Could you check a few things on this model? Use its own coordinates, in mm. Give positions to 0.01 mm unless a question says otherwise; leave off trailing zeros. Loops run counter-clockwise (first coordinate to the right, second up) from the corner with the lowest first, then second, coordinate; pieces in that order, holes last. Notation, with made-up numbers: (42, 23.25) -> (68, 23.25) arc R12 cw to (68, 29.25) -> close; hole circle Ø6 at (88.25, 23.25). An arc over 180 degrees is marked (long way). Write item = value, one per line. Start each with the question number.
1) I want a section at B-B (x = 35). List the corners of the cut face in (y, z) for me.
2) I'm going to push flat-ended pins straight in: pin 1 Ø4 at (y, z) = (167.5, 12) entering from +X; pin 2 Ø10 at (x, y) = (14.5, 78.5) entering from -Z; pin 3 Ø3 at (y, z) = (142.5, 20) entering from -X. Where does each tip first touch, or does it pass through?
3) I want a section at C-C (y = 74.5). List the corners of the cut face in (x, z) for me, and give its area (3 significant figures).
4) If we mould it in two halves opening along X, with no side actions, what happens to faces 1 (the face through (-10.84, 98.6, 48.81)), 2 (the face through (-34, 0, 33)), 3 (the face through (-21.68, 144.19, -42.03))? For each: +X half, -X half, draft (parallel to the pull), parting line (faces both ways), or undercut.
5) I want a section at A-A (z = 0). List the corners of the cut face in (x, y) for me.
6) I need wall thicknesses on probe 1 along X at (y, z) = (125, 0); probe 2 along Z at (x, y) = (0, 144). Which ranges of each line are inside material? Lowest first, please. Write a range as from..to.
from build123d import *

# Parameters (mm, degrees)
EXTRUDE_1_OUTLINE_R      = 50
EXTRUDE_1_OUTLINE_R_2    = 47
EXTRUDE_1_DEPTH          = 200
CUT_EXTRUDE_1_DEPTH      = 213.132034356
CUT_EXTRUDE_1_DEPTH_BACK = 213.132034356
SKETCH_2_R               = 66.5


# Read off the part's stored shape, not the designer's step: Вытянуть-Тонкостенный1
with BuildPart() as part:
    # Вытянуть-Тонкостенный1 outline → Вытянуть-Тонкостенный1 (new body)
    with BuildSketch(Plane(origin=(0, 0, 0), x_dir=(1, 0, 0), z_dir=(0, 1, 0))):
        Circle(EXTRUDE_1_OUTLINE_R)
        Circle(EXTRUDE_1_OUTLINE_R_2, mode=Mode.SUBTRACT)
    extrude(amount=EXTRUDE_1_DEPTH)

    # Эскиз2 → Вырез-Вытянуть1 (cut, two sides: drawn at the far end of the back side and taken through both)
    with BuildSketch(Plane(origin=(0, 0, 0), x_dir=(1, 0, 0), z_dir=(0, -0.819152044288991, -0.5735764363510473)).offset(-CUT_EXTRUDE_1_DEPTH_BACK)):
        with Locations((0, -180)):
            Circle(SKETCH_2_R)
    extrude(amount=CUT_EXTRUDE_1_DEPTH + CUT_EXTRUDE_1_DEPTH_BACK, mode=Mode.SUBTRACT)


solid = part.part
Answer list:
q1.outline = (0, -35.71) -> (164.24, -35.71) -> (170.44, -31.37) -> (0, -31.37) -> close; (0, 31.37) -> (200, 31.37) -> (200, 35.71) -> (0, 35.71) -> close
q2.pin_1 = 48.99
q2.pin_2 = -49.09
q2.pin_3 = -46.45
q3.outline = circle Ø100 at (0, 0); hole circle Ø94 at (0, 0)
q3.area = 914 mm^2
q4.face_1 = parting line
q4.face_2 = draft
q4.face_3 = undercut
q5.outline = (-50, 0) -> (-47, 0) -> (-47, 200) -> (-50, 200) -> close; (47, 0) -> (50, 0) -> (50, 200) -> (47, 200) -> close
q6.probe_1 = -50..-47, 47..50
q6.probe_2 = 47..50
